Read the model definition and answer for the solid it produces. Units are mm, in the model's axes. A direction names the side the tool comes from. Round coordinates to 2 decimals unless told otherwise and drop trailing zeros. Loops run counter-clockwise (first coordinate to the right, second up) from the corner with the lowest first, then second, coordinate; pieces in that order, holes last. Notation, with made-up numbers: (30, 44.25) - (68, 44.25) arc R21 ccw to (68, 75.25) - close; hole circle Ø1 at (15.5, 44). An arc over 180 degrees is marked (long way). Answer as CSV lines item,"result".
```python
from build123d import *

# Parameters (mm, degrees)
F0_R     = 34.5
F0_R_2   = 34
F0_R_3   = 33.5
F1_DEPTH = 5
F2_DEPTH = 19
F4_SIZE  = 3


with BuildPart() as f1:
    # F0 (on Top) → F1 (new body)
    with BuildSketch(Plane.XY):
        Circle(F0_R)
        Circle(F0_R_2, mode=Mode.SUBTRACT)
        Circle(F0_R_2)
        Circle(F0_R_3, mode=Mode.SUBTRACT)
        Circle(F0_R_3)
    extrude(amount=F1_DEPTH)

    # F0 (on Top) → F2 (join)
    with BuildSketch(Plane.XY):
        Circle(F0_R_3)
    extrude(amount=-F2_DEPTH)

    # F4
    f4_edges = [f1.edges().sort_by_distance(p)[0] for p in [
        (-33.5, 0, -19),
    ]]
    chamfer(f4_edges, length=F4_SIZE)


solid = f1.part
```
1) Find the intervals of material crossed by line 1 (Z direction, x = -6, y = -30); line 2 (Y direction, x = -29, z = 1.5); line 3 (Y direction, x = 1.5, z = -9.5), in increasing order.
Entries:
line 1,"z = -18.91 to 5"
line 2,"y = -18.69 to 18.69"
line 3,"y = -33.47 to 33.47"
2) A cutting plane is placed at A-A, the plane x = 0. Determine the outline of the cut face in (y, z), plus the area to 3 significant figures.
Entries:
outline,"(-34.5, 0) - (-33.5, 0) - (-33.5, -16) - (-30.5, -19) - (30.5, -19) - (33.5, -16) - (33.5, 0) - (34.5, 0) - (34.5, 5) - (-34.5, 5) - close"
area,"1,610 mm^2"
3) A cutting plane is placed at D-D, the plane z = 2.25. Determine the outline of the cut face in (x, y), plus the area to 3 significant figures.
Entries:
outline,"circle Ø69 at (0, 0)"
area,"3,740 mm^2"
4) A cutting plane is placed at C-C, the plane z = -9.75. Determine the outline of the cut face in (x, y), plus the area to 3 significant figures.
Entries:
outline,"circle Ø67 at (0, 0)"
area,"3,530 mm^2"
5) The mould has two halves that part along Z. Classify faces 1 (the face through (0, 0, 5)), 2 (the face through (-7.262, -32.703, -7.888)), 3 (the face through (-6.64, -29.92, -18.85)): pulls with the +Z half, pulls with the -Z half, needs draft (parallel to the pull), parting line crosses it, or undercut.
Entries:
face 1,"pulls with the +Z half"
face 2,"needs draft"
face 3,"pulls with the -Z half"
6) Each of these flat-tipped pins is pushed along its axis until it touches: P1, Ø10, axis at x = -14.5, z = -14.5, coming from the +Y side; P2, Ø4, axis at x = -5, z = 2, coming from the +Y side; P3, Ø8, axis at y = 1, z = -14, coming from the +X side. Where does it stop, or does it pass through?
Entries:
P1,"stops at y = 32.12"
P2,"stops at y = 34.37"
P3,"stops at x = 33.5"
7) A tool of negligible diameter and unlimited length cuts with its end or side. For faces 4 (the face through (-5.3, 33.4, 0)), 5 (the face through (32.907, 10.363, 2.465)), from which of +Z, -Z, +X, -X, +Y, -Y can it reach the whole face along a straight path? Write none if from no direction.
Entries:
face 4,"-Z"
face 5,"+Z, -Z"
